Verification items for the finished model (mm, model axes). Face numbers are marked on the shaded views. A direction names the side the tool comes from. Coordinates: 2 decimals unless noted, no trailing zeros. Loops run counter-clockwise (first coordinate to the right, second up) from the corner with the lowest first, then second, coordinate; pieces in that order, holes last. Notation, with made-up numbers: (11.5, 71.5) - (55.5, 71.5) arc R19 cw to (55.5, 86.5) - close; hole circle Ø6 at (-17, 30). An arc over 180 degrees is marked (long way). Answer as CSV lines item,"result". Start each with the question number.
1. Cross-section at C-C (z = -4.5). Enter the section's corners in (x, y).
2. Material ranges on line 1 (Y direction, x = -11.25, z = 1); line 2 (X direction, y = -23.5, z = -9); line 3 (Y direction, x = -1.3, z = 0), recorded low to high. Write a range as [from, to].
3. Cross-section at B-B (x = -18). Enter the section's corners in (y, z).
4. Cross-section at A-A (z = 0). Enter the section's corners in (x, y).
5. Cross-section at D-D (y = -25). Enter the section's corners in (x, z), plus the area to 3 significant figures.
6. Set-up check for the marked faces 1 and 2: record each of +Z, -Z, +X, -X, +Y, -Y from which the full face is reachable in a straight line by a thin tool's end or side.
7. Gauge pin test, flat ends, axial feed: P1, Ø10, axis at x = -6.5, z = 13.5, coming from the +Y side; P2, Ø20, axis at y = 14, z = 9.5, coming from the -X side; P3, Ø7.5, axis at x = -17, z = 4.5, coming from the -Y side; P4, Ø1.5, axis at x = -6.5, z = -15, coming from the -Y side. Record the tip position at first contact, or that the pin passes through.
```python
from build123d import *

# Parameters (mm, degrees)
SKETCH1_W                    = 40
SKETCH1_H                    = 100
BASE_FLANGE1_DEPTH           = 5
EDGE_FLANGE1_STRIP_W         = 26
EDGE_FLANGE1_STRIP_H         = 5
EDGE_FLANGE1_STRIP_CUT_DEPTH = 40
EDGE_FLANGE1_DEPTH           = 40
SKETCH9_R                    = 2.5
CUT_EXTRUDE1_DEPTH           = 10
FILLET1_R                    = 10
SKETCH16_R                   = 3
CUT_EXTRUDE2_DEPTH           = 10


# Sheet-metal steps are written as plain solids
with BuildPart() as part:
    # Sketch1 → Base-Flange1 (new body)
    with BuildSketch(Plane(origin=(0, 0, 0), x_dir=(0, 0, -1), z_dir=(1, 0, 0))):
        Rectangle(SKETCH1_W, SKETCH1_H)
    extrude(amount=-BASE_FLANGE1_DEPTH)

    # Edge-Flange1 strip (across the edge) → Edge-Flange1 strip cut (cut)
    with BuildSketch(Plane(origin=(-5, 50, 20), x_dir=(0, -1, 0), z_dir=(0, 0, -1))):
        with Locations((-5, -2.5)):
            Rectangle(EDGE_FLANGE1_STRIP_W, EDGE_FLANGE1_STRIP_H)
    extrude(amount=EDGE_FLANGE1_STRIP_CUT_DEPTH, mode=Mode.SUBTRACT)

    # Edge-Flange1 section (across the edge) → Edge-Flange1 (add)
    with BuildSketch(Plane(origin=(-5, 50, 20), x_dir=(0, -1, 0), z_dir=(0, 0, -1))):
        with BuildLine():
            Line((0, 3), (0, 18))
            Line((0, 18), (5, 18))
            Line((5, 18), (5, 3))
            ThreePointArc((5, 3), (5.878679656, 0.878679656), (8, 0))
            Line((8, 0), (8, -5))
            ThreePointArc((8, -5), (2.343145751, -2.656854249), (0, 3))
        make_face()
    extrude(amount=EDGE_FLANGE1_DEPTH)

    # Sketch9 → Cut-Extrude1 (cut)
    with BuildSketch(Plane(origin=(0, 50, 0), x_dir=(1, 0, 0), z_dir=(0, 1, 0))):
        with Locations(Location((-18, 10, 0), (0, 0, 180))):
            Circle(SKETCH9_R)
        with Locations(Location((-18, -10, 0), (0, 0, 180))):
            Circle(SKETCH9_R)
    extrude(amount=-CUT_EXTRUDE1_DEPTH, mode=Mode.SUBTRACT)

    # Fillet1
    fillet1_edges = [part.edges().sort_by_distance(p)[0] for p in [
        (-23, 47.5, 20),
        (-23, 47.5, -20),
        (-2.5, -50, -20),
        (-2.5, -50, 20),
    ]]
    fillet(fillet1_edges, radius=FILLET1_R)

    # Sketch16 → Cut-Extrude2 (cut)
    with BuildSketch(Plane(origin=(0, 0, 0), x_dir=(0, 0, -1), z_dir=(1, 0, 0))):
        Circle(SKETCH16_R)
        with Locations((0, -30)):
            Circle(SKETCH16_R)
        with Locations((0, 25)):
            Circle(SKETCH16_R)
    extrude(amount=-CUT_EXTRUDE2_DEPTH, mode=Mode.SUBTRACT)


solid = part.part
```
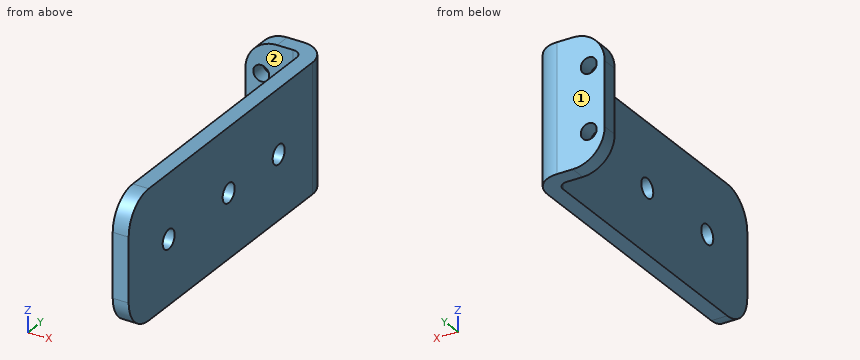
Values follow:
1,outline,"(-23, 45) - (-8, 45) arc R3 cw to (-5, 42) - (-5, -50) - (0, -50) - (0, 42) arc R8 ccw to (-8, 50) - (-23, 50) - close"
2,line 1,"y = [45, 50]"
2,line 2,"x = [-5, 0]"
2,line 3,"y = [-50, -33], [-27, -3], [3, 22], [28, 46.37]"
3,outline,"(45, -18.66) - (50, -18.66) - (50, -12.5) - (45, -12.5) - close; (45, -7.5) - (50, -7.5) - (50, 7.5) - (45, 7.5) - close; (45, 12.5) - (50, 12.5) - (50, 18.66) - (45, 18.66) - close"
4,outline,"(-23, 45) - (-8, 45) arc R3 cw to (-5, 42) - (-5, 28) - (0, 28) - (0, 42) arc R8 ccw to (-8, 50) - (-23, 50) - close; (-5, -50) - (0, -50) - (0, -33) - (-5, -33) - close; (-5, -27) - (0, -27) - (0, -3) - (-5, -3) - close; (-5, 3) - (0, 3) - (0, 22) - (-5, 22) - close"
5,outline,"(-5, -20) - (0, -20) - (0, 20) - (-5, 20) - close"
5,area,"200 mm²"
6,face 1,"+Z, -Z, +X, -X, +Y"
6,face 2,"+Z, -Z, -X, -Y"
7,P1,"stops at y = 50"
7,P2,"stops at x = -5"
7,P3,"stops at y = 45"
7,P4,"stops at y = 43.98"
